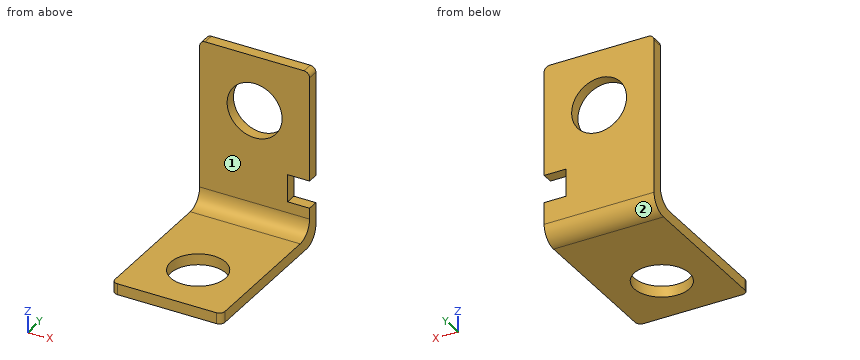
from build123d import *

# Parameters (mm, degrees)
F0_R     = 5
F1_DEPTH = 2
F2_W     = 20
F2_H     = 2
F3_DEPTH = 30
F4_R     = 3
F5_R     = 5
F6_DEPTH = 2.001
F7_R     = 1


with BuildPart() as f1:
    # F0 (on Front) → F1 (new body)
    with BuildSketch(Plane.XZ):
        Polygon((10, 15), (-10, 15), (-10, -15), (10, -15), (10, -10), (6, -10), (6, -5), (10, -5), align=None)
        with Locations((0, 5)):
            Circle(F0_R, mode=Mode.SUBTRACT)
    extrude(amount=F1_DEPTH)

    # F2 (on face) → F3 (join)
    with BuildSketch(Plane(origin=(0, 0, 0), x_dir=(-1, 0, 0), z_dir=(0, 1, 0))):
        with Locations((0, -16)):
            Rectangle(F2_W, F2_H)
    extrude(amount=-F3_DEPTH)

    # F4
    f4_edges = [f1.edges().sort_by_distance(p)[0] for p in [
        (0, -2, -15),
        (0, 0, -17),
    ]]
    fillet(f4_edges, radius=F4_R)

    # F5 (on face) → F6 (cut, through all)
    with BuildSketch(Plane.XY.offset(-15)):
        with Locations((0, -20)):
            Circle(F5_R)
    extrude(amount=-F6_DEPTH, mode=Mode.SUBTRACT)

    # F7
    f7_edges = [f1.edges().sort_by_distance(p)[0] for p in [
        (-10, -1, 15),
        (10, -1, 15),
        (-10, -30, -16),
        (10, -30, -16),
    ]]
    fillet(f7_edges, radius=F7_R)


solid = f1.part
For this review, take the finished solid that the model builds, in its own axes (mm). Face numbers are marked on the shaded views. A direction names the side the tool comes from. Give positions to 0.01 mm unless a question says otherwise; leave off trailing zeros. Loops run counter-clockwise (first coordinate to the right, second up) from the corner with the lowest first, then second, coordinate; pieces in that order, holes last. Notation, with made-up numbers: (8.25, 7) -> (28.25, 7) arc R7 cw to (28.25, 19) -> close; hole circle Ø1 at (-32.75, -12.5). An arc over 180 degrees is marked (long way). One line per question, with ' | ' between items.
1) We need section B-B (y = -20). Write out the cut boundary in (x, z), plus the area to 3 significant figures.
Resolved:
outline: (-10, -17) -> (-5, -17) -> (-5, -15) -> (-10, -15) -> close; (5, -17) -> (10, -17) -> (10, -15) -> (5, -15) -> close | area: 20.0 mm2
2) For the marked faces 1 and 2, list the 3-axis set-ups (+Z, -Z, +X, -X, +Y, -Y) from which the entire face can be reached by the end or side of a thin tool; tool diameter is ignored.
Resolved:
face 1: +Z, +X, -X, -Y | face 2: -Z, +X, -X, +Y
3) We need section C-C (z = 5). Write out the cut boundary in (x, y), plus the area to 3 significant figures.
Resolved:
outline: (-10, -2) -> (-5, -2) -> (-5, 0) -> (-10, 0) -> close; (5, -2) -> (10, -2) -> (10, 0) -> (5, 0) -> close | area: 20.0 mm2
4) We need section A-A (x = 0). Write out the cut boundary in (y, z), plus the area to 3 significant figures.
Resolved:
outline: (-30, -17) -> (-25, -17) -> (-25, -15) -> (-30, -15) -> close; (-15, -17) -> (-3, -17) arc R3 ccw to (0, -14) -> (0, 0) -> (-2, 0) -> (-2, -12) arc R3 cw to (-5, -15) -> (-15, -15) -> close; (-2, 10) -> (0, 10) -> (0, 15) -> (-2, 15) -> close | area: 80.0 mm2
5) To check wall thickness, follow probe 1 along Y at (x, z) = (-1, 12); probe 2 along Z at (x, y) = (5.5, -18.5); probe 3 along Y at (x, z) = (0, -15.9). State the ranges of each line that lie inside material, in increasing order.
Resolved:
probe 1: y = -2 to 0 | probe 2: z = -17 to -15 | probe 3: y = -30 to -25, -15 to -0.68
6) Insertion check: pin 1 Ø10 at (y, z) = (-11.5, -9.5) entering from -X; pin 2 Ø6 at (x, z) = (2, 0.5) entering from -Y; pin 3 Ø10 at (x, z) = (1, -9) entering from -Y; pin 4 Ø1.6 at (y, z) = (-1, -7.5) entering from +X. Each pin has a flat end and moves straight along its axis. Give the tip position at first contact, or say it passes through.
Resolved:
pin 1: passes through | pin 2: stops at y = -2 | pin 3: stops at y = -2.76 | pin 4: stops at x = 6
7) We need section D-D (x = 4.5). Write out the cut boundary in (y, z).
Resolved:
outline: (-30, -17) -> (-22.18, -17) -> (-22.18, -15) -> (-30, -15) -> close; (-17.82, -17) -> (-3, -17) arc R3 ccw to (0, -14) -> (0, 2.82) -> (-2, 2.82) -> (-2, -12) arc R3 cw to (-5, -15) -> (-17.82, -15) -> close; (-2, 7.18) -> (0, 7.18) -> (0, 15) -> (-2, 15) -> close
